Design review of the part shown in the three views and the two pictorial views. Dimensions are in mm from the part's minimum x, y and z. Give positions to 0.01 mm unless a question says otherwise; leave off trailing zeros. Order: outer loops, then holes, each group sorted by start corner. A loop starts at its lowest first (then second) coordinate and runs counter-clockwise, first axis right, second up.
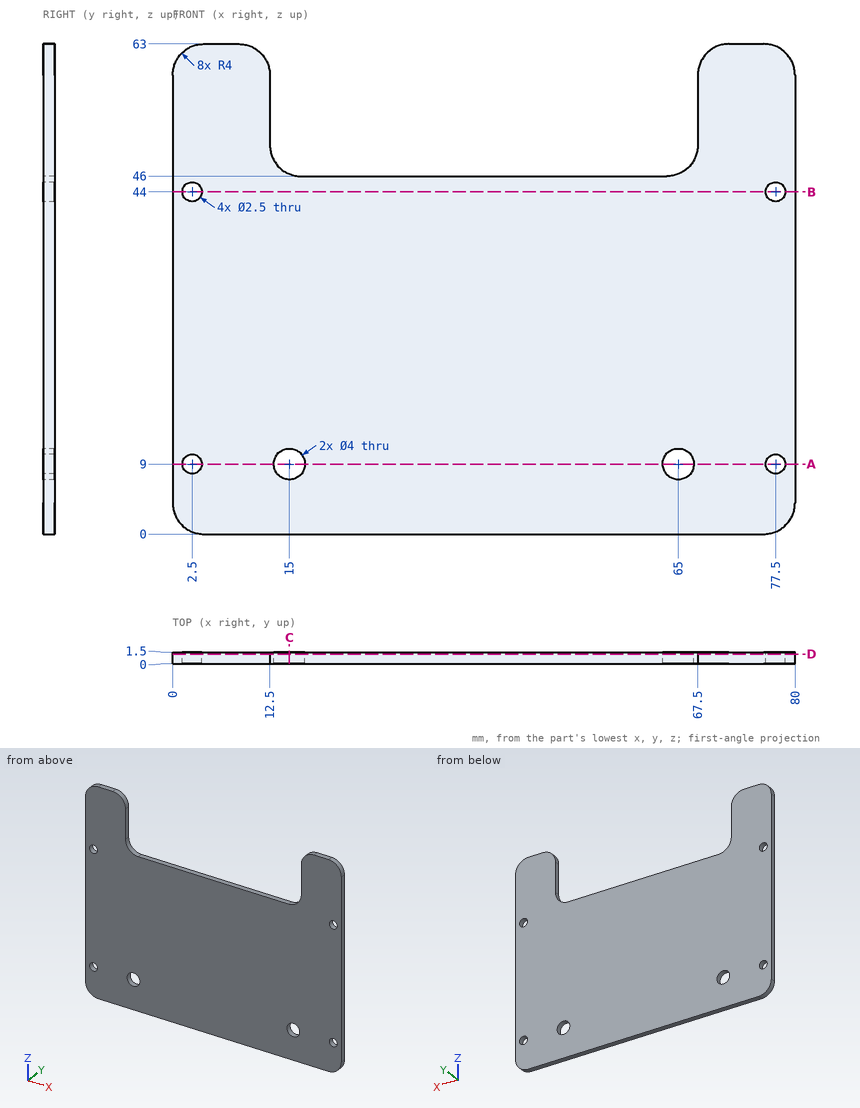
Item 1: For line 1 (Z direction, x = 77.5, y = 0.4); line 2 (Z direction, x = 49, y = 1.4); line 3 (Z direction, x = 3, y = 0.45), list the stretches that pass through material, from the lowest coordinate up.
Values found:
line 1: z = 0.29 to 7.75, 10.25 to 42.75, 45.25 to 62.71
line 2: z = 0 to 46
line 3: z = 0.13 to 7.85, 10.15 to 42.85, 45.15 to 62.87
Item 2: Take a section at B-B (z = 44). Give the boundary of the cut face in (x, y), and give its area (4 significant figures).
Values found:
outline: (0, 0) - (1.25, 0) - (1.25, 1.5) - (0, 1.5) - close; (3.75, 0) - (76.25, 0) - (76.25, 1.5) - (3.75, 1.5) - close; (78.75, 0) - (80, 0) - (80, 1.5) - (78.75, 1.5) - close
area: 112.5 mm2
Item 3: Take a section at D-D (y = 1.25). Give the boundary of the cut face in (x, z).
Values found:
outline: (0, 4) arc R4 ccw to (4, 0) - (76, 0) arc R4 ccw to (80, 4) - (80, 59) arc R4 ccw to (76, 63) - (71.5, 63) arc R4 ccw to (67.5, 59) - (67.5, 50) arc R4 cw to (63.5, 46) - (16.5, 46) arc R4 cw to (12.5, 50) - (12.5, 59) arc R4 ccw to (8.5, 63) - (4, 63) arc R4 ccw to (0, 59) - close; hole circle Ø2.5 at (2.5, 9); hole circle Ø2.5 at (2.5, 44); hole circle Ø4 at (15, 9); hole circle Ø4 at (65, 9); hole circle Ø2.5 at (77.5, 9); hole circle Ø2.5 at (77.5, 44)
Item 4: Take a section at A-A (z = 9). Give the boundary of the cut face in (x, y).
Values found:
outline: (0, 0) - (1.25, 0) - (1.25, 1.5) - (0, 1.5) - close; (3.75, 0) - (13, 0) - (13, 1.5) - (3.75, 1.5) - close; (17, 0) - (63, 0) - (63, 1.5) - (17, 1.5) - close; (67, 0) - (76.25, 0) - (76.25, 1.5) - (67, 1.5) - close; (78.75, 0) - (80, 0) - (80, 1.5) - (78.75, 1.5) - close
Item 5: Take a section at C-C (x = 15). Give the boundary of the cut face in (y, z).
Values found:
outline: (0, 0) - (1.5, 0) - (1.5, 7) - (0, 7) - close; (0, 11) - (1.5, 11) - (1.5, 46.29) - (0, 46.29) - close
Item 6: Clearance check with a flat-ended pin moving along its axis: pin 1 Ø3 at (x, z) = (15, 9) entering from -Y. State where the tip first meets the part, or that it passes through.
Values found:
pin 1: passes through
